For this review, take the finished solid that the model builds, in its own axes (mm). Face numbers are marked on the shaded views. Coordinates: 2 decimals unless noted, no trailing zeros. Loops run counter-clockwise (first coordinate to the right, second up) from the corner with the lowest first, then second, coordinate; pieces in that order, holes last. Notation, with made-up numbers: (23, 58) -> (38, 58) arc R11 ccw to (38, 65) -> close; hole circle Ø3 at (75.25, 14.5). An arc over 180 degrees is marked (long way). One line per item, written item: value.
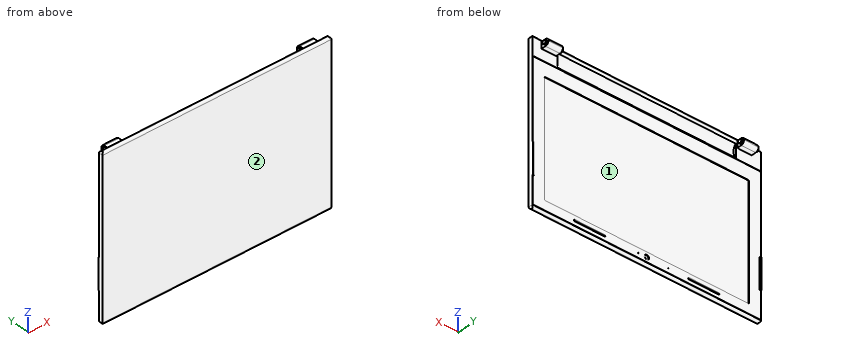
from build123d import *

# Parameters (mm, degrees)
SKETCH1_W            = 380
SKETCH1_H            = 265
BOSS_EXTRUDE1_DEPTH  = 7
FILLET2_R            = 3.5
BOSS_EXTRUDE2_DEPTH  = 0.5
CUT_EXTRUDE1_DEPTH   = 1
SKETCH4_R            = 4
CUT_EXTRUDE2_DEPTH   = 1
SKETCH5_R            = 0.625
CUT_EXTRUDE3_DEPTH   = 1
SKETCH6_R            = 0.625
CUT_EXTRUDE4_DEPTH   = 1
SKETCH7_W            = 24
SKETCH7_H            = 10.979763194
BOSS_EXTRUDE3_DEPTH  = 13
CUT_EXTRUDE6_DEPTH   = 27
SKETCH9_R            = 3
BOSS_EXTRUDE4_DEPTH  = 2.5
BOSS_EXTRUDE5_START  = 2.5
SKETCH10_R           = 3
BOSS_EXTRUDE5_DEPTH  = 2.5
SKETCH11_W           = 24
SKETCH11_H           = 10.98
BOSS_EXTRUDE6_DEPTH  = 13
CUT_EXTRUDE9_DEPTH   = 296
SKETCH22_R           = 3
BOSS_EXTRUDE7_DEPTH  = 2.5
BOSS_EXTRUDE8_START  = 2.5
SKETCH23_R           = 3
BOSS_EXTRUDE8_DEPTH  = 2.5
CUT_EXTRUDE10_DEPTH  = 296
DRAFT1_ANGLE         = 20
DRAFT2_ANGLE         = 20
BOSS_EXTRUDE9_DEPTH  = 1
SKETCH33_R           = 2
BOSS_EXTRUDE10_DEPTH = 0.5


with BuildPart() as part:
    # Sketch1 → Boss-Extrude1 (new body)
    with BuildSketch(Plane(origin=(0, 0, 0), x_dir=(1, 0, 0), z_dir=(0, 1, 0))):
        with Locations((190, -132.5)):
            Rectangle(SKETCH1_W, SKETCH1_H)
    extrude(amount=BOSS_EXTRUDE1_DEPTH)

    # Fillet2
    fillet2_edges = [part.edges().sort_by_distance(p)[0] for p in [
        (190, 7, 0),
        (190, 0, 0),
        (190, 0, 265),
        (190, 7, 265),
        (0, 3.5, 0),
        (380, 3.5, 0),
        (380, 3.5, 265),
        (0, 3.5, 265),
    ]]
    fillet(fillet2_edges, radius=FILLET2_R - 0.0001)  # a hair under: the kernel refuses the full size

    # Sketch2 → Boss-Extrude2 (add)
    with BuildSketch(Plane(origin=(0, 7, 0), x_dir=(1, 0, 0), z_dir=(0, 1, 0))):
        with BuildLine():
            Line((1.25, -3.75), (378.75, -3.75))
            ThreePointArc((378.75, -3.75), (379.457106781, -4.042893219), (379.75, -4.75))
            Line((379.75, -4.75), (379.75, -232.5))
            ThreePointArc((379.75, -232.5), (379.457106781, -233.207106781), (378.75, -233.5))
            Line((378.75, -233.5), (1.25, -233.5))
            ThreePointArc((1.25, -233.5), (0.542893219, -233.207106781), (0.25, -232.5))
            Line((0.25, -232.5), (0.25, -4.75))
            ThreePointArc((0.25, -4.75), (0.542893219, -4.042893219), (1.25, -3.75))
        make_face()
        with BuildLine():
            Line((2.25, -4.75), (377.75, -4.75))
            ThreePointArc((377.75, -4.75), (378.457106781, -5.042893219), (378.75, -5.75))
            Line((378.75, -5.75), (378.75, -231.5))
            ThreePointArc((378.75, -231.5), (378.457106781, -232.207106781), (377.75, -232.5))
            Line((377.75, -232.5), (2.25, -232.5))
            ThreePointArc((2.25, -232.5), (1.542893219, -232.207106781), (1.25, -231.5))
            Line((1.25, -231.5), (1.25, -5.75))
            ThreePointArc((1.25, -5.75), (1.542893219, -5.042893219), (2.25, -4.75))
        make_face(mode=Mode.SUBTRACT)
    extrude(amount=BOSS_EXTRUDE2_DEPTH)

    # Sketch3 → Cut-Extrude1 (cut)
    with BuildSketch(Plane(origin=(0, 7, 0), x_dir=(1, 0, 0), z_dir=(0, 1, 0))):
        with BuildLine():
            Line((21.5, -20), (358.5, -20))
            ThreePointArc((358.5, -20), (359.560660172, -20.439339828), (360, -21.5))
            Line((360, -21.5), (360, -208.5))
            ThreePointArc((360, -208.5), (359.560660172, -209.560660172), (358.5, -210))
            Line((358.5, -210), (21.5, -210))
            ThreePointArc((21.5, -210), (20.439339828, -209.560660172), (20, -208.5))
            Line((20, -208.5), (20, -21.5))
            ThreePointArc((20, -21.5), (20.439339828, -20.439339828), (21.5, -20))
        make_face()
    extrude(amount=-CUT_EXTRUDE1_DEPTH, mode=Mode.SUBTRACT)

    # Sketch4 → Cut-Extrude2 (cut)
    with BuildSketch(Plane(origin=(0, 7, 0), x_dir=(1, 0, 0), z_dir=(0, 1, 0))):
        with Locations(Location((190, -11.584908102, 0), (0, 0, 270))):
            Circle(SKETCH4_R)
    extrude(amount=-CUT_EXTRUDE2_DEPTH, mode=Mode.SUBTRACT)

    # Sketch5 → Cut-Extrude3 (cut)
    with BuildSketch(Plane(origin=(0, 7, 0), x_dir=(1, 0, 0), z_dir=(0, 1, 0))):
        with Locations(Location((154.376617555, -11.584908102, 0), (0, 0, 270))):
            Circle(SKETCH5_R)
    extrude(amount=-CUT_EXTRUDE3_DEPTH, mode=Mode.SUBTRACT)

    # Sketch6 → Cut-Extrude4 (cut)
    with BuildSketch(Plane(origin=(0, 7, 0), x_dir=(1, 0, 0), z_dir=(0, 1, 0))):
        with Locations(Location((204.109733731, -11.584908102, 0), (0, 0, 270))):
            Circle(SKETCH6_R)
    extrude(amount=-CUT_EXTRUDE4_DEPTH, mode=Mode.SUBTRACT)

    # Sketch7 → Boss-Extrude3 (add)
    with BuildSketch(Plane(origin=(0, 7, 0), x_dir=(1, 0, 0), z_dir=(0, 1, 0))):
        with Locations((27.5, -256.010118403)):
            Rectangle(SKETCH7_W, SKETCH7_H)
    extrude(amount=BOSS_EXTRUDE3_DEPTH)

    # Sketch8 → Cut-Extrude6 (cut)
    with BuildSketch(Plane.ZY.offset(-15.5)):
        with BuildLine():
            Line((250.520236806, 20), (250.520236806, 14.510118403))
            ThreePointArc((250.520236806, 14.510118403), (252.128185898, 18.392050908), (256.010118403, 20))
            Line((256.010118403, 20), (250.520236806, 20))
        make_face()
        with BuildLine():
            Line((261.5, 20), (256.010118403, 20))
            ThreePointArc((256.010118403, 20), (259.892050908, 18.392050908), (261.5, 14.510118403))
            Line((261.5, 14.510118403), (261.5, 20))
        make_face()
    extrude(amount=-CUT_EXTRUDE6_DEPTH, mode=Mode.SUBTRACT)

    # Sketch9 → Boss-Extrude4 (add)
    with BuildSketch(Plane.ZY.offset(-15.5)):
        with Locations(Location((256.010118403, 14.510118403, 0), (0, 0, 180))):
            Circle(SKETCH9_R)
    extrude(amount=BOSS_EXTRUDE4_DEPTH)

    # Sketch10 → Boss-Extrude5 (add)
    with BuildSketch(Plane(origin=(39.5, 0, 0), x_dir=(0, 0, -1), z_dir=(1, 0, 0)).offset(BOSS_EXTRUDE5_START)):
        with Locations((-256.010118403, 14.510118403)):
            Circle(SKETCH10_R)
    extrude(amount=-BOSS_EXTRUDE5_DEPTH)

    # Sketch11 → Boss-Extrude6 (add)
    with BuildSketch(Plane(origin=(0, 7, 0), x_dir=(1, 0, 0), z_dir=(0, 1, 0))):
        with Locations((352.5, -256.01)):
            Rectangle(SKETCH11_W, SKETCH11_H)
    extrude(amount=BOSS_EXTRUDE6_DEPTH)

    # Sketch21 → Cut-Extrude9 (cut)
    with BuildSketch(Plane(origin=(364.5, 0, 0), x_dir=(0, 0, -1), z_dir=(1, 0, 0))):
        with BuildLine():
            Line((-250.52, 20), (-256.01, 20))
            ThreePointArc((-256.01, 20), (-252.127983771, 18.392016229), (-250.52, 14.51))
            Line((-250.52, 14.51), (-250.52, 20))
        make_face()
        with BuildLine():
            Line((-261.5, 20), (-261.5, 14.51))
            ThreePointArc((-261.5, 14.51), (-259.892016229, 18.392016229), (-256.01, 20))
            Line((-256.01, 20), (-261.5, 20))
        make_face()
    extrude(amount=-CUT_EXTRUDE9_DEPTH, mode=Mode.SUBTRACT)

    # Sketch22 → Boss-Extrude7 (add)
    with BuildSketch(Plane(origin=(364.5, 0, 0), x_dir=(0, 0, -1), z_dir=(1, 0, 0))):
        with Locations(Location((-256.01, 14.51, 0), (0, 0, 180))):
            Circle(SKETCH22_R)
    extrude(amount=BOSS_EXTRUDE7_DEPTH)

    # Sketch23 → Boss-Extrude8 (add)
    with BuildSketch(Plane.ZY.offset(-340.5).offset(BOSS_EXTRUDE8_START)):
        with Locations((256.01, 14.51)):
            Circle(SKETCH23_R)
    extrude(amount=-BOSS_EXTRUDE8_DEPTH)

    # Sketch31 → Cut-Extrude10 (cut)
    with BuildSketch(Plane(origin=(42, 0, 0), x_dir=(0, 0, -1), z_dir=(1, 0, 0))):
        with BuildLine():
            Line((-256.010118403, 7), (-234.010118403, 7))
            ThreePointArc((-234.010118403, 7), (-245.010118403, 3.88854382), (-256.010118403, 7))
        make_face()
    extrude(amount=CUT_EXTRUDE10_DEPTH, mode=Mode.SUBTRACT)

    # Draft1
    draft1_faces = [part.faces().sort_by_distance(p)[0] for p in [
        (338, 5.747159877, 245.010118403),
    ]]
    draft(draft1_faces, Plane.ZX.offset(7), DRAFT1_ANGLE)

    # Draft2
    draft2_faces = [part.faces().sort_by_distance(p)[0] for p in [
        (42, 5.747159877, 245.010118403),
    ]]
    draft(draft2_faces, Plane.ZX.offset(7), DRAFT2_ANGLE)

    # Sketch32 → Boss-Extrude9 (add)
    with BuildSketch(Plane(origin=(0, 7, 0), x_dir=(1, 0, 0), z_dir=(0, 1, 0))):
        with BuildLine():
            Line((70, -10.584908102), (120, -10.584908102))
            ThreePointArc((120, -10.584908102), (121, -11.584908102), (120, -12.584908102))
            Line((120, -12.584908102), (70, -12.584908102))
            ThreePointArc((70, -12.584908102), (69, -11.584908102), (70, -10.584908102))
        make_face()
        with BuildLine():
            Line((260, -10.881099807), (310, -10.881099807))
            ThreePointArc((310, -10.881099807), (311, -11.881099807), (310, -12.881099807))
            Line((310, -12.881099807), (260, -12.881099807))
            ThreePointArc((260, -12.881099807), (259, -11.881099807), (260, -10.881099807))
        make_face()
        with BuildLine():
            Line((2.25, -50), (2.25, -100))
            ThreePointArc((2.25, -100), (1.25, -101), (0.25, -100))
            Line((0.25, -100), (0.25, -50))
            ThreePointArc((0.25, -50), (1.25, -49), (2.25, -50))
        make_face()
        with BuildLine():
            Line((379.75, -50), (379.75, -100))
            ThreePointArc((379.75, -100), (378.75, -101), (377.75, -100))
            Line((377.75, -100), (377.75, -50))
            ThreePointArc((377.75, -50), (378.75, -49), (379.75, -50))
        make_face()
    extrude(amount=BOSS_EXTRUDE9_DEPTH)

    # Sketch33 → Boss-Extrude10 (add)
    with BuildSketch(Plane(origin=(0, 6, 0), x_dir=(1, 0, 0), z_dir=(0, 1, 0))):
        with Locations(Location((190, -11.584908102, 0), (0, 0, 270))):
            Circle(SKETCH33_R)
    extrude(amount=BOSS_EXTRUDE10_DEPTH)


solid = part.part
1. Take a section at C-C, the plane z = 88. Give the boundary of the cut face in (x, y), and give its area (3 significant figures).
Return value:
outline: (0, 0) -> (380, 0) -> (380, 7) -> (379.75, 7) -> (379.75, 8) -> (377.75, 8) -> (377.75, 7) -> (360, 7) -> (360, 6) -> (20, 6) -> (20, 7) -> (2.25, 7) -> (2.25, 8) -> (0.25, 8) -> (0.25, 7) -> (0, 7) -> close
area: 2,320 mm2
2. To check wall thickness, follow probe 1 along Z at (x, y) = (277.5, 6.5); probe 2 along Y at (x, z) = (349.5, 60); probe 3 along Y at (x, z) = (26.5, 11). State the ranges of each line that lie inside material, in increasing order. Write a range as from..to.
Return value:
probe 1: z = 1.7..20, 210..234.87, 255.15..263.3
probe 2: y = 0..6
probe 3: y = 0..7
3. Take a section at A-A, the plane z = 173.5. Give the boundary of the cut face in (x, y), and give its area (3 significant figures).
Return value:
outline: (0, 0) -> (380, 0) -> (380, 7) -> (379.75, 7) -> (379.75, 7.5) -> (378.75, 7.5) -> (378.75, 7) -> (360, 7) -> (360, 6) -> (20, 6) -> (20, 7) -> (1.25, 7) -> (1.25, 7.5) -> (0.25, 7.5) -> (0.25, 7) -> (0, 7) -> close
area: 2,320 mm2
4. Insertion check: pin 1 Ø6.5 at (x, z) = (188.5, 13.5) entering from +Y; pin 2 Ø0.5 at (y, z) = (7.5, 166.5) entering from +X; pin 3 Ø5.5 at (y, z) = (11.5, 258.5) entering from -X. Each pin has a flat end and moves straight along its axis. Give the tip position at first contact, or say it passes through.
Return value:
pin 1: stops at y = 7
pin 2: stops at x = 379.75
pin 3: stops at x = 13
5. The part is to be moulded in two halves that separate along X. For the marked faces 1 and 2, say which applies: pulls with the +X half, pulls with the -X half, needs draft (parallel to the pull), parting line crosses it, or undercut.
Return value:
face 1: undercut
face 2: needs draft
